Build history of the part. All positions in model axes, mm. A direction names the side the tool comes from. Give positions to 0.01 mm unless a question says otherwise; leave off trailing zeros. Loops run counter-clockwise (first coordinate to the right, second up) from the corner with the lowest first, then second, coordinate; pieces in that order, holes last. Notation, with made-up numbers: M 6,56 L 26,56 A20 cw 26,75 Z; hole C -28,19 d6. An arc over 180 degrees is marked long. Answer as a JSON object with one key per item and string values. Group by question number.
1. Slice it at A-A (z = 0). List the corners of the cut face in (x, y), then the cut area to 3 significant figures.
2. Drill centre lines: line 1 along Y through (x, z) = (1.5, 0); line 2 along Z through (x, y) = (0.75, 51); line 3 along Z through (x, y) = (-3.5, 104). Where is each one in solid material? Low to high. Write a range as [from, to].
3. 3-axis set-ups, long thin cutter, end or side, ignore diameter. For faces 4 (the face through (-3.3, 0, -1.2)), 5 (the face through (0, 17, 0)): which of +Z, -Z, +X, -X, +Y, -Y reach the whole face in a straight line?
4. Slice it at C-C (y = 108). List the corners of the cut face in (x, z).
5. Drop flat-ended pins along their axis: pin 1 Ø3 at (y, z) = (95.5, 3) entering from +X; pin 2 Ø5 at (y, z) = (18.5, 3.5) entering from +X; pin 3 Ø1 at (x, y) = (-2, 63) entering from -Z. Give the stop position or say it passes through.
6. Mould opens along Z. For faces 1 (the face through (0.73, 8.62, 3.27)), 2 (the face through (0, 120, 0)), 3 (the face through (-4.88, 59.16, -1.08)) say: released by +Z, released by -Z, zero draft, split by the parting line, or undercut.
7. Slice it at B-B (x = 0). List the corners of the cut face in (y, z), then the cut area to 3 significant figures.
from build123d import *

# Parameters (mm, degrees)
SKETCH4_R           = 5
BOSS_EXTRUDE1_DEPTH = 120
SKETCH5_W           = 3.35
SKETCH5_H           = 17


with BuildPart() as part:
    # Sketch3 → Revolve1 (revolve)
    with BuildSketch(Plane.XY, mode=Mode.PRIVATE) as revolve1_sk:
        Polygon((0, 0), (2.7, 0), (3.35, 17), (0, 17), align=None)
    revolve(revolve1_sk.sketch.rotate(Axis((0, 17, 0), (0, -1, 0)), 180), axis=Axis((0, 17, 0), (0, -1, 0)))

    # Sketch4 → Boss-Extrude1 (add)
    with BuildSketch(Plane(origin=(0, 0, 0), x_dir=(1, 0, 0), z_dir=(0, 1, 0))):
        with Locations(Location((0, 0, 0), (0, 0, 270))):
            Circle(SKETCH4_R)
    extrude(amount=BOSS_EXTRUDE1_DEPTH)

    # Sketch5 → Cut-Revolve1 (revolve, cut)
    with BuildSketch(Plane.XY, mode=Mode.PRIVATE) as cut_revolve1_sk:
        with Locations((1.675, 8.5)):
            Rectangle(SKETCH5_W, SKETCH5_H)
    revolve(cut_revolve1_sk.sketch.rotate(Axis((0, 17, 0), (0, -1, 0)), 180), axis=Axis((0, 17, 0), (0, -1, 0)), mode=Mode.SUBTRACT)


solid = part.part
Established:
{
 "1": {"outline": "M -5,0 L -3.35,0 L -3.35,17 L 3.35,17 L 3.35,0 L 5,0 L 5,120 L -5,120 Z", "area": "1,090 mm^2"},
 "2": {"line 1": "y = [17, 120]", "line 2": "z = [-4.94, 4.94]", "line 3": "z = [-3.57, 3.57]"},
 "3": {"face 4": "+Z, -Z, +X, -X, -Y", "face 5": "-Y"},
 "4": {"outline": "C 0,0 d10"},
 "5": {"pin 1": "stops at x = 4.77", "pin 2": "stops at x = 4.9", "pin 3": "stops at z = -4.77"},
 "6": {"face 1": "undercut", "face 2": "zero draft", "face 3": "split by the parting line"},
 "7": {"outline": "M 0,-5 L 120,-5 L 120,5 L 0,5 L 0,3.35 L 17,3.35 L 17,-3.35 L 0,-3.35 Z", "area": "1,090 mm^2"}
}
